from build123d import *

# Parameters (mm, degrees)
SKETCH1_W           = 1310.386
SKETCH1_H           = 101.6
BOSS_EXTRUDE1_DEPTH = 69.85
BOSS_EXTRUDE2_DEPTH = 68.326
SKETCH3_W           = 79.430838384
SKETCH3_H           = 176.27
BOSS_EXTRUDE3_DEPTH = 76.23
SKETCH4_W           = 146.04
SKETCH4_H           = 156.04
BOSS_EXTRUDE4_DEPTH = 146.05
SKETCH5_R           = 28.575
CUT_EXTRUDE1_DEPTH  = 927.1


with BuildPart() as part:
    # Sketch1 → Boss-Extrude1 (new, symmetric)
    with BuildSketch(Plane(origin=(0, 0, 0), x_dir=(0, 0, -1), z_dir=(1, 0, 0))):
        with Locations((-655.193, 0)):
            Rectangle(SKETCH1_W, SKETCH1_H)
    extrude(amount=BOSS_EXTRUDE1_DEPTH, both=True)

    # Sketch2 → Boss-Extrude2 (add, symmetric)
    with BuildSketch(Plane(origin=(0, 0, 0), x_dir=(0, 0, -1), z_dir=(1, 0, 0))):
        Polygon((0, 0), (0, -68.326), (79.430838384, -68.326), (79.430838384, 85.598), (0, 85.598), align=None)
    extrude(amount=BOSS_EXTRUDE2_DEPTH, both=True)

    # Sketch3 → Boss-Extrude3 (add, symmetric)
    with BuildSketch(Plane(origin=(0, 0, 0), x_dir=(0, 0, -1), z_dir=(1, 0, 0))):
        with Locations((39.715419192, 173.733)):
            Rectangle(SKETCH3_W, SKETCH3_H)
    extrude(amount=BOSS_EXTRUDE3_DEPTH, both=True)

    # Sketch4 → Boss-Extrude4 (add)
    with BuildSketch(Plane.XY):
        with Locations((1.79, 173.848)):
            Rectangle(SKETCH4_W, SKETCH4_H)
    extrude(amount=BOSS_EXTRUDE4_DEPTH)

    # Sketch5 → Cut-Extrude1 (cut)
    with BuildSketch(Plane.XY.offset(1310.386)):
        Circle(SKETCH5_R)
    extrude(amount=-CUT_EXTRUDE1_DEPTH, mode=Mode.SUBTRACT)


solid = part.part
The listing builds one solid part. Answer for the finished solid, in the listing's coordinates (mm). A direction names the side the tool comes from. Coordinates: 2 decimals unless noted, no trailing zeros. Write each loop counter-clockwise with the first axis right and the second up, starting at its lowest first coordinate (ties: lowest second). Pieces come first, ordered by that corner, then holes. Notation, with made-up numbers: (47.5, 62) - (82.5, 62) arc R15 ccw to (82.5, 73) - close; hole circle Ø9 at (40, -10.5). An arc over 180 degrees is marked (long way). Put each result on its own line as item: value.
1. A tool of negligible diameter and unlimited length cuts with its end or side. For faces 5 (the face through (74.81, 173, 72)), 6 (the face through (1, -68.326, -39)), 7 (the face through (1, 251.868, 72)), 8 (the face through (1, -50.8, 664)), 9 (the face through (1, 94, -79.431)), from which of +Z, -Z, +X, -X, +Y, -Y can it reach the whole face along a straight path? Write none if from no direction.
Answer sheet:
face 5: +Z, +X, +Y, -Y
face 6: +Z, -Z, +X, -X, -Y
face 7: +Z, +X, -X, +Y
face 8: +Z, +X, -X, -Y
face 9: -Z, +X, -X, +Y, -Y
2. Flat-ended cylindrical pins translate along their axes: pin 1 Ø0.5 at (x, y) = (69, 16) entering from -Z; pin 2 Ø2.5 at (x, z) = (-74, -35.5) entering from -Y; pin 3 Ø2 at (x, z) = (3.5, 342) entering from +Y; pin 4 Ø6.5 at (x, z) = (71.5, -49.5) entering from -Y. Find the tip coordinate at first contact, or state that the pin passes through.
Answer sheet:
pin 1: stops at z = 0
pin 2: stops at y = 85.6
pin 3: stops at y = 50.8
pin 4: stops at y = -68.33
3. The part is cut by section C-C on z = 620. Give the vertices of the cut face in (x, y) (3 decimals).
Answer sheet:
outline: (-69.85, -50.8) - (69.85, -50.8) - (69.85, 50.8) - (-69.85, 50.8) - close; hole circle Ø57.15 at (0, 0)
4. The part is cut by section D-D on y = 149. Give the vertices of the cut face in (x, z).
Answer sheet:
outline: (-76.23, -79.43) - (76.23, -79.43) - (76.23, 0) - (74.81, 0) - (74.81, 146.05) - (-71.23, 146.05) - (-71.23, 0) - (-76.23, 0) - close
5. The part is cut by section A-A on y = 0. Give the vertices of the cut face in (x, z) (3 decimals).
Answer sheet:
outline: (-69.85, 0) - (-68.326, 0) - (-68.326, -79.431) - (68.326, -79.431) - (68.326, 0) - (69.85, 0) - (69.85, 1310.386) - (28.575, 1310.386) - (28.575, 383.286) - (-28.575, 383.286) - (-28.575, 1310.386) - (-69.85, 1310.386) - close
6. Find the intervals of material crossed by line 1 along Y through (x, z) = (0, 583.5) (3 decimals); line 2 along Y through (x, z) = (35, 483); line 3 along Z through (x, y) = (12, 97.5), in increasing order. Write a range as from..to.
Answer sheet:
line 1: y = -50.8..-28.575, 28.575..50.8
line 2: y = -50.8..50.8
line 3: z = -79.43..146.05
7. Determine the mould class of faces 1 (the face through (-68.326, 10, -39)), 2 (the face through (-28.547, 1.256, 853.326)), 3 (the face through (1, 95.828, 72)), 4 (the face through (68.326, 10, -39)) for opening direction X: pulls with the +X half, pulls with the -X half, needs draft (parallel to the pull), parting line crosses it, or undercut.
Answer sheet:
face 1: pulls with the -X half
face 2: undercut
face 3: needs draft
face 4: pulls with the +X half
8. The part is cut by section B-B on x = 0. Give the vertices of the cut face in (y, z) (3 decimals), plus the area to 3 significant figures.
Answer sheet:
outline: (-68.326, -79.431) - (261.868, -79.431) - (261.868, 0) - (251.868, 0) - (251.868, 146.05) - (95.828, 146.05) - (95.828, 0) - (50.8, 0) - (50.8, 1310.386) - (28.575, 1310.386) - (28.575, 383.286) - (-28.575, 383.286) - (-28.575, 1310.386) - (-50.8, 1310.386) - (-50.8, 0) - (-68.326, 0) - close
area: 129,000 mm^2
